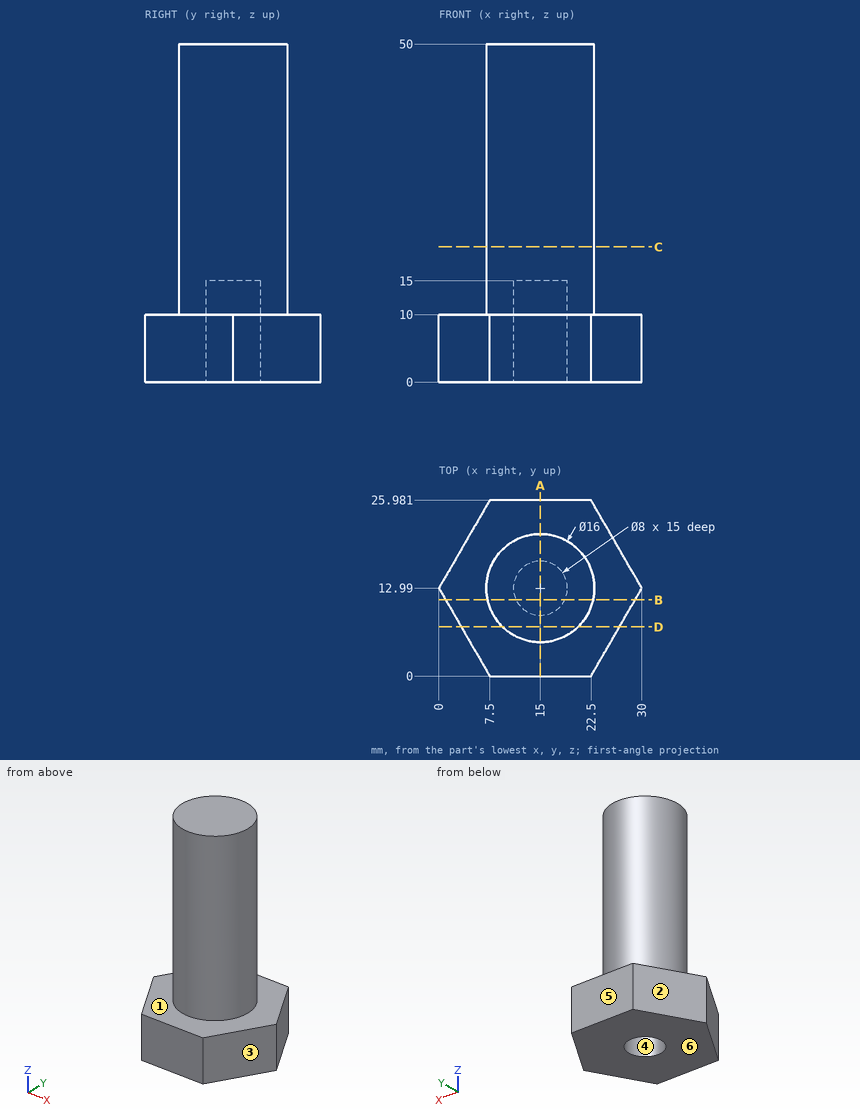
Study the drawing (mm; zero at the part's minimum x, y, z) and answer. A direction names the side the tool comes from. Give positions to 0.01 mm unless a question says otherwise; leave off trailing zeros. Loops run counter-clockwise (first coordinate to the right, second up) from the corner with the lowest first, then second, coordinate; pieces in that order, holes last. Notation, with made-up numbers: (76.5, 6) - (121.5, 6) arc R22 cw to (121.5, 25) - close; hole circle Ø3 at (13, -11). An arc over 180 degrees is marked (long way). Answer as CSV lines item,"result". Start each with the question number.
1) Find section A-A (x = 15). Write down the section's boundary in (y, z), then the cut area to 3 significant figures.
2) Each of these flat-tipped pins is pushed along its axis until it touches: pin 1 Ø2 at (y, z) = (15.5, 18.5) entering from +X; pin 2 Ø5 at (x, y) = (15, 12.99) entering from -Z; pin 3 Ø4 at (x, z) = (25.5, 41) entering from -Y; pin 4 Ø1.5 at (x, z) = (12.5, 39) entering from -Y. Where does it stop, or does it pass through?
3) Find section B-B (y = 11.25). Write down the section's boundary in (x, z) (1 decimal).
4) Straight lines are drawn through the part: L1, parallel to Y at x = 15, z = 9.25; L2, parallel to Y at x = 15, z = 11.5; L3, parallel to Z at x = 5.5, y = 7.25. For each, find the intervals that lie inside material, in ascending order. Write a range as from..to.
5) Find section C-C (z = 20). Write down the section's boundary in (x, y).
6) Determine the mould class of the marked faces 3, 4, 5 and 6 for opening direction Y: released by +Y, released by -Y, zero draft, split by the parting line, or undercut.
7) Which of the six approach directions +Z, -Z, +X, -X, +Y, -Y give full straight-line access (tool end or side, diameter ignored) to the marked faces 1 and 2?
8) Find section D-D (y = 7.25). Write down the section's boundary in (x, z).
Findings below:
1,outline,"(0, 0) - (8.99, 0) - (8.99, 15) - (16.99, 15) - (16.99, 0) - (25.98, 0) - (25.98, 10) - (20.99, 10) - (20.99, 50) - (4.99, 50) - (4.99, 10) - (0, 10) - close"
1,area,"780 mm^2"
2,pin 1,"x = 22.86"
2,pin 2,"z = 15"
2,pin 3,"through"
2,pin 4,"y = 5.18"
3,outline,"(1, 0) - (11.4, 0) - (11.4, 15) - (18.6, 15) - (18.6, 0) - (29, 0) - (29, 10) - (22.8, 10) - (22.8, 50) - (7.2, 50) - (7.2, 10) - (1, 10) - close"
4,L1,"0..8.99, 16.99..25.98"
4,L2,"4.99..8.99, 16.99..20.99"
4,L3,"0..10"
5,outline,"circle Ø16 at (15, 12.99)"
6,face 3,"released by -Y"
6,face 4,"undercut"
6,face 5,"released by +Y"
6,face 6,"zero draft"
7,face 1,"+Z"
7,face 2,"+Z, -Z, -X, +Y"
8,outline,"(3.31, 0) - (26.69, 0) - (26.69, 10) - (20.57, 10) - (20.57, 50) - (9.43, 50) - (9.43, 10) - (3.31, 10) - close"
